Verification items for this drawing (mm, ordinates from the low corner). A direction names the side the tool comes from. Round coordinates to 2 decimals unless told otherwise and drop trailing zeros. Order: outer loops, then holes, each group sorted by start corner. A loop starts at its lowest first (then second) coordinate and runs counter-clockwise, first axis right, second up. Notation, with made-up numbers: (55.25, 50.5) - (101.25, 50.5) arc R22 ccw to (101.25, 63.5) - close; hole circle Ø10 at (-36, 24). An arc over 180 degrees is marked (long way). Return JSON: item names as keys, results as strings. Group by question number.
Q1. Sectioned sample at D-D, the plane y = 12.75. Record the cut outline in (x, z), then the cut area to 3 significant figures.
Q2. Gauge pin test, flat ends, axial feed: pin 1 Ø1 at (x, z) = (11.5, 5) entering from +Y; pin 2 Ø1 at (x, z) = (4, 1.5) entering from -Y; pin 3 Ø1 at (y, z) = (5.5, 7) entering from +X; pin 4 Ø1.5 at (x, y) = (10, 10) entering from -Z. Record the tip position at first contact, or that the pin passes through.
Q3. Sectioned sample at C-C, the plane z = 6.75. Record the cut outline in (x, y), then the cut area to 3 significant figures.
Q4. Material ranges on line 1 along Y through (x, z) = (10, 3.25); line 2 along Y through (x, z) = (10, 6); line 3 along Z through (x, y) = (4, 2.75), recorded low to high.
Q5. Tool access check on the marked faces 1 and 2. Record the directions out of +Z, -Z, +X, -X, +Y, -Y that give a thin tool (end or side, any length) a straight path to the whole face; none if there is none.
Q6. Sectioned sample at A-A, the plane x = 10. Record the cut outline in (y, z), then the cut area to 3 significant figures.
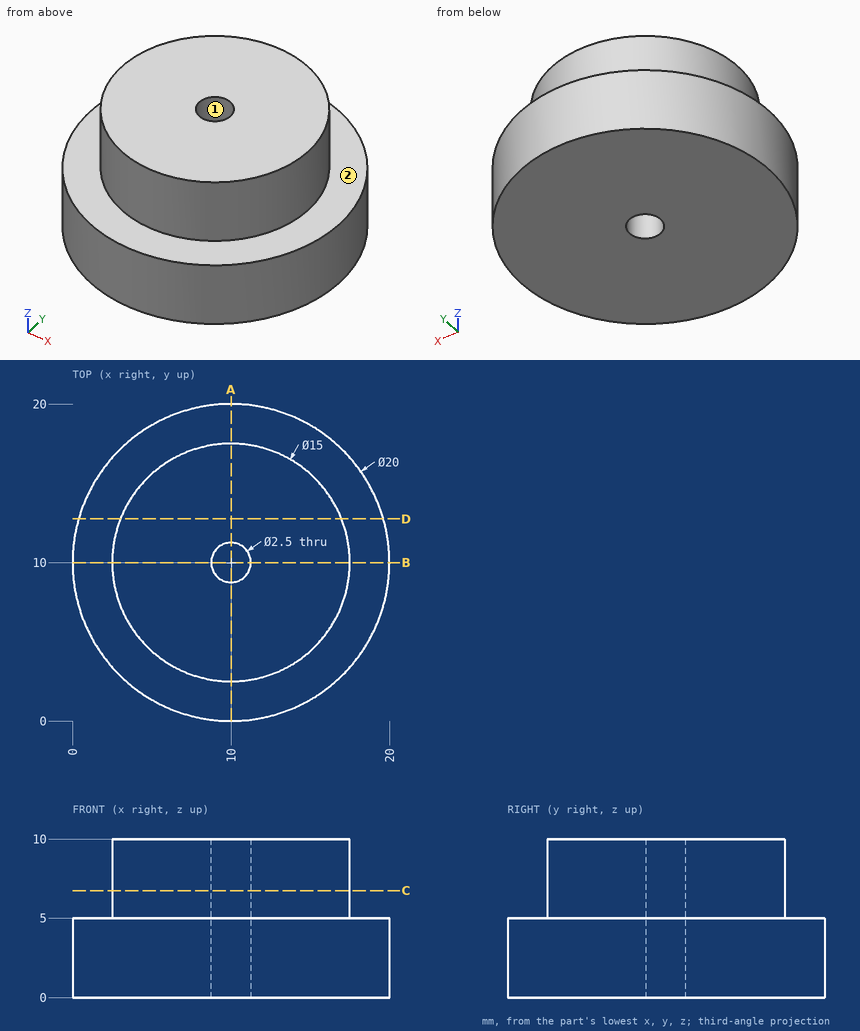
Reply:
{
 "1": {"outline": "(0.39, 0) - (19.61, 0) - (19.61, 5) - (16.98, 5) - (16.98, 10) - (3.02, 10) - (3.02, 5) - (0.39, 5) - close", "area": "166 mm^2"},
 "2": {"pin 1": "y = 19.95", "pin 2": "y = 1.65", "pin 3": "x = 16.34", "pin 4": "through"},
 "3": {"outline": "circle Ø15 at (10, 10); hole circle Ø2.5 at (10, 10)", "area": "172 mm^2"},
 "4": {"line 1": "0 to 8.75, 11.25 to 20", "line 2": "2.5 to 8.75, 11.25 to 17.5", "line 3": "0 to 5"},
 "5": {"face 1": "+Z, -Z", "face 2": "+Z"},
 "6": {"outline": "(0, 0) - (8.75, 0) - (8.75, 10) - (2.5, 10) - (2.5, 5) - (0, 5) - close; (11.25, 0) - (20, 0) - (20, 5) - (17.5, 5) - (17.5, 10) - (11.25, 10) - close", "area": "150 mm^2"}
}
